The listing builds one solid part. Answer for the finished solid, in the listing's coordinates (mm). A direction names the side the tool comes from. Give positions to 0.01 mm unless a question says otherwise; leave off trailing zeros. Loops run counter-clockwise (first coordinate to the right, second up) from the corner with the lowest first, then second, coordinate; pieces in that order, holes last.
Item 1: This flat-tipped pin is pushed along its axis until it touches: pin 1 Ø10 at (x, z) = (-27.5, -15) entering from +Y. Where does it stop, or does it pass through?
Item 2: Consider line 1 along X through (y, z) = (4, -13.5); line 2 along Z through (x, y) = (-23, 42); line 3 along Y through (x, z) = (41.5, -9.5). Determine where each line is inside the solid, lowest interval first.
Item 3: Section B-B, the plane z = 19 is taken. Give the vertices of the cut face in (x, y).
Item 4: Section C-C, the plane x = -11 is taken. Give the vertices of the cut face in (y, z).
Item 5: A tool of negligible diameter and unlimited length cuts with its end or side. For faces 1 (the face through (0, 46.5, 0)), 2 (the face through (-1, 0, 0)), from which of +Z, -Z, +X, -X, +Y, -Y can it reach the whole face along a straight path? Write none if from no direction.
Item 6: The mould has two halves that part along Z. Classify faces 3 (the face through (-1, 25, -30)), 4 (the face through (-45, 25, 0)), 5 (the face through (0.75, 24, 15)): pulls with the +Z half, pulls with the -Z half, needs draft (parallel to the pull), parting line crosses it, or undercut.
Item 7: Section A-A, the plane y = 39.5 is taken. Give the vertices of the cut face in (x, z), and give its area (3 significant figures).
from build123d import *

# Parameters (mm, degrees)
SKETCH_1_W      = 87
SKETCH_1_H      = 57
EXTRUDE_1_DEPTH = 1.5
SKETCH_1_3_W    = 90
SKETCH_1_3_H    = 60
SKETCH_1_3_W_2  = 87
SKETCH_1_3_H_2  = 57
EXTRUDE_2_DEPTH = 50
EXTRUDE_3_DEPTH = 45


with BuildPart() as part:
    # 草图1 → 凸台-拉伸1 (new body)
    with BuildSketch(Plane(origin=(0, 0, 0), x_dir=(1, 0, 0), z_dir=(0, 1, 0))):
        Rectangle(SKETCH_1_W, SKETCH_1_H)
    extrude(amount=EXTRUDE_1_DEPTH)

    # 草图1<3> → 凸台-拉伸2 (add)
    with BuildSketch(Plane(origin=(0, 0, 0), x_dir=(1, 0, 0), z_dir=(0, 1, 0))):
        Rectangle(SKETCH_1_3_W, SKETCH_1_3_H)
        Rectangle(SKETCH_1_3_W_2, SKETCH_1_3_H_2, mode=Mode.SUBTRACT)
    extrude(amount=EXTRUDE_2_DEPTH)

    # 草图2 → 凸台-拉伸3 (add)
    with BuildSketch(Plane(origin=(0, 1.5, 0), x_dir=(1, 0, 0), z_dir=(0, 1, 0))):
        Polygon((0.75, -0.75), (43.5, -0.75), (43.5, 0.75), (0.75, 0.75), (0.75, 28.5), (-0.75, 28.5), (-0.75, 0.75), (-43.5, 0.75), (-43.5, -0.75), (-0.75, -0.75), (-0.75, -28.5), (0.75, -28.5), align=None)
    extrude(amount=EXTRUDE_3_DEPTH)


solid = part.part
Worked answers:
1. pin 1: stops at y = 1.5
2. line 1: x = -45 to -43.5, -0.75 to 0.75, 43.5 to 45
2. line 2: z = -30 to -28.5, -0.75 to 0.75, 28.5 to 30
2. line 3: y = 0 to 1.5
3. outline: (-45, 0) - (45, 0) - (45, 50) - (43.5, 50) - (43.5, 1.5) - (0.75, 1.5) - (0.75, 46.5) - (-0.75, 46.5) - (-0.75, 1.5) - (-43.5, 1.5) - (-43.5, 50) - (-45, 50) - close
4. outline: (0, -30) - (50, -30) - (50, -28.5) - (1.5, -28.5) - (1.5, -0.75) - (46.5, -0.75) - (46.5, 0.75) - (1.5, 0.75) - (1.5, 28.5) - (50, 28.5) - (50, 30) - (0, 30) - close
5. face 1: +Y
5. face 2: +Z, -Z, +X, -X, -Y
6. face 3: pulls with the -Z half
6. face 4: needs draft
6. face 5: undercut
7. outline: (-45, -30) - (45, -30) - (45, 30) - (-45, 30) - close; hole (-43.5, -28.5) - (-0.75, -28.5) - (-0.75, -0.75) - (-43.5, -0.75) - close; hole (-43.5, 0.75) - (-0.75, 0.75) - (-0.75, 28.5) - (-43.5, 28.5) - close; hole (0.75, -28.5) - (43.5, -28.5) - (43.5, -0.75) - (0.75, -0.75) - close; hole (0.75, 0.75) - (43.5, 0.75) - (43.5, 28.5) - (0.75, 28.5) - close
7. area: 655 mm2
